Geometry check sheet. Reference: the model listing, model coordinates, mm. Face numbers are marked on the shaded views. A direction names the side the tool comes from. Round coordinates to 2 decimals unless told otherwise and drop trailing zeros. Loops run counter-clockwise (first coordinate to the right, second up) from the corner with the lowest first, then second, coordinate; pieces in that order, holes last. Notation, with made-up numbers: M 12,-20 L 31,-20 A18 ccw 31,-6 Z; hole C -20.5,55.5 d8. An arc over 180 degrees is marked long. Write item = value, one per line.
from build123d import *

# Parameters (mm, degrees)
F0_W          = 5.2
F0_H          = 10
F1_DEPTH      = 16
F0_H_2        = 40
F2_DEPTH      = 10.5
F3_R          = 3.25
F4_DEPTH      = 25
F4_DEPTH_BACK = 62.6
F5_DEPTH      = 5
F5_DEPTH_BACK = 45
F6_R          = 2.5
F7_DEPTH      = 20
F8_R          = 3


with BuildPart() as f1:
    # F0 (on Top) → F1 (new body)
    with BuildSketch(Plane.XY):
        with Locations((-13.1, 25)):
            Rectangle(F0_W, F0_H)
        Polygon((-15.7, -30), (-15.7, -20), (-15.7, 20), (-15.7, 30), (-20, 30), (-20, -30), align=None)
        with Locations((-13.1, -25)):
            Rectangle(F0_W, F0_H)
        Polygon((10, -30), (10.5, -30), (10.5, -20), (-10.5, -20), (-10.5, -30), (-10, -30), align=None)
        with Locations((13.1, -25)):
            Rectangle(F0_W, F0_H)
        Polygon((15.7, -30), (20, -30), (20, 30), (15.7, 30), (15.7, 20), (15.7, -20), align=None)
        with Locations((13.1, 25)):
            Rectangle(F0_W, F0_H)
        Polygon((10.5, 20), (10.5, 30), (10, 30), (-10, 30), (-10.5, 30), (-10.5, 20), align=None)
    extrude(amount=F1_DEPTH)

    # F0 (on Top) → F2 (join)
    with BuildSketch(Plane.XY):
        with Locations((-13.1, 0)):
            Rectangle(F0_W, F0_H_2)
        with Locations((13.1, 0)):
            Rectangle(F0_W, F0_H_2)
    extrude(amount=F2_DEPTH)

    # F3 (on face) → F4 (cut, two sides)
    with BuildSketch(Plane(origin=(0, -20, 0), x_dir=(-1, 0, 0), z_dir=(0, 1, 0))) as f4_sk:
        with Locations((0, 7.6108775102)):
            Circle(F3_R)
    extrude(amount=-F4_DEPTH, mode=Mode.SUBTRACT)
    extrude(f4_sk.sketch, amount=F4_DEPTH_BACK, mode=Mode.SUBTRACT)

    # F3 (on face) → F5 (cut, two sides)
    with BuildSketch(Plane(origin=(0, -20, 0), x_dir=(-1, 0, 0), z_dir=(0, 1, 0))) as f5_sk:
        Polygon((-2.9280820296, 12.7203134505), (-5.8889423381, 7.6298020583), (-2.9608603085, 2.520366118), (2.9280820296, 2.5014415699), (5.8889423381, 7.591952962), (2.9608603085, 12.7013889023), align=None)
        with Locations((0, 7.6108775102)):
            Circle(F3_R, mode=Mode.SUBTRACT)
    extrude(amount=-F5_DEPTH, mode=Mode.SUBTRACT)
    extrude(f5_sk.sketch, amount=F5_DEPTH_BACK, mode=Mode.SUBTRACT)

    # F6 (on face) → F7 (cut)
    with BuildSketch(Plane.XY.offset(16)):
        with Locations((-15, -25)):
            Circle(F6_R)
        with Locations((15, -25)):
            Circle(F6_R)
        with Locations((15, 25)):
            Circle(F6_R)
        with Locations((-15, 25)):
            Circle(F6_R)
    extrude(amount=-F7_DEPTH, mode=Mode.SUBTRACT)

    # F8
    f8_edges = [f1.edges().sort_by_distance(p)[0] for p in [
        (20, -30, 8),
        (20, 30, 8),
        (-20, 30, 8),
        (-20, -30, 8),
    ]]
    fillet(f8_edges, radius=F8_R)


solid = f1.part
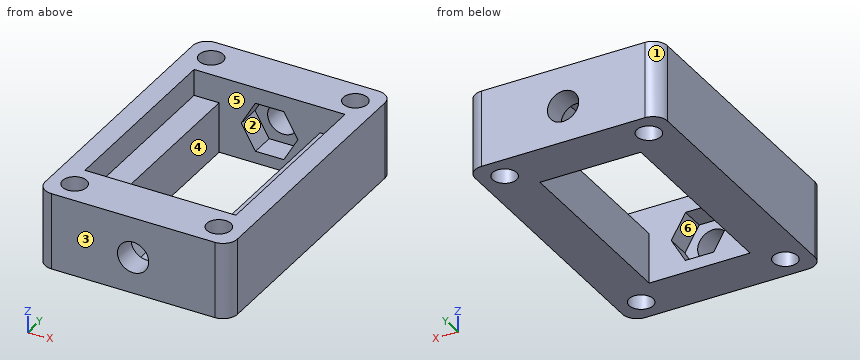
(1) Sectioned sample at B-B on y = 3. Record the cut outline in (x, z), then the cut area to 3 significant figures.
Result set:
outline = M -20,0 L -10.5,0 L -10.5,10.5 L -15.7,10.5 L -15.7,16 L -20,16 Z; M 10.5,0 L 20,0 L 20,16 L 15.7,16 L 15.7,10.5 L 10.5,10.5 Z
area = 247 mm2
(2) Tool access check on the marked faces 4, 5 and 6. Record the directions out of +Z, -Z, +X, -X, +Y, -Y that give a thin tool (end or side, any length) a straight path to the whole face; none if there is none.
Result set:
face_4 = +Z, -Z
face_5 = +Z
face_6 = none
(3) Sectioned sample at D-D on z = 14. Record the cut outline in (x, y).
Result set:
outline = M -20,-27 A3 ccw -17,-30 L 17,-30 A3 ccw 20,-27 L 20,27 A3 ccw 17,30 L -17,30 A3 ccw -20,27 Z; hole C -15,-25 d5; hole C -15,25 d5; hole M -15.7,-20 L 15.7,-20 L 15.7,20 L -15.7,20 Z; hole C 15,-25 d5; hole C 15,25 d5
(4) Release check for a two-part mould opening along Y. For the marked faces 1, 2 and 3 record: released by +Y, released by -Y, zero draft, split by the parting line, or undercut.
Result set:
face_1 = released by +Y
face_2 = undercut
face_3 = released by -Y
(5) Material ranges on line 1 along Y through (x, z) = (15, 4.5); line 2 along Z through (x, y) = (0, 26); line 3 along X through (y, z) = (-9, 3.5), recorded low to high. Write a range as from..to.
Result set:
line_1 = -30..-27.5, -22.5..22.5, 27.5..30
line_2 = 0..4.36, 10.86..16
line_3 = -20..-10.5, 10.5..20
(6) Sectioned sample at A-A on x = 15. Record the cut outline in (y, z).
Result set:
outline = M -30,0 L -27.5,0 L -27.5,16 L -30,16 Z; M -22.5,0 L 22.5,0 L 22.5,16 L 20,16 L 20,10.5 L -20,10.5 L -20,16 L -22.5,16 Z; M 27.5,0 L 30,0 L 30,16 L 27.5,16 Z
(7) Depth check by flat-ended pin: pin 1 Ø12 at (x, y) = (-2, 8.5) entering from -Z; pin 2 Ø3 at (x, z) = (2, 8) entering from +Y. Enter the tip coordinate at first touch or a pass-through.
Result set:
pin_1 = through
pin_2 = 30
(8) Sectioned sample at C-C on x = -9.5. Record the cut outline in (y, z), then the cut area to 3 significant figures.
Result set:
outline = M -30,0 L -20,0 L -20,16 L -30,16 Z; M 20,0 L 30,0 L 30,16 L 20,16 Z
area = 320 mm2
